Geometry check sheet. Reference: drawing and pictorial views, mm from the part's lowest x, y, z. A direction names the side the tool comes from. Round coordinates to 2 decimals unless told otherwise and drop trailing zeros. Loops run counter-clockwise (first coordinate to the right, second up) from the corner with the lowest first, then second, coordinate; pieces in that order, holes last. Notation, with made-up numbers: (37, -10) - (51, -10) arc R34 cw to (51, 20) - close; hole circle Ø2 at (33, 76.5). An arc over 180 degrees is marked (long way). Return JSON: item names as keys, results as strings.
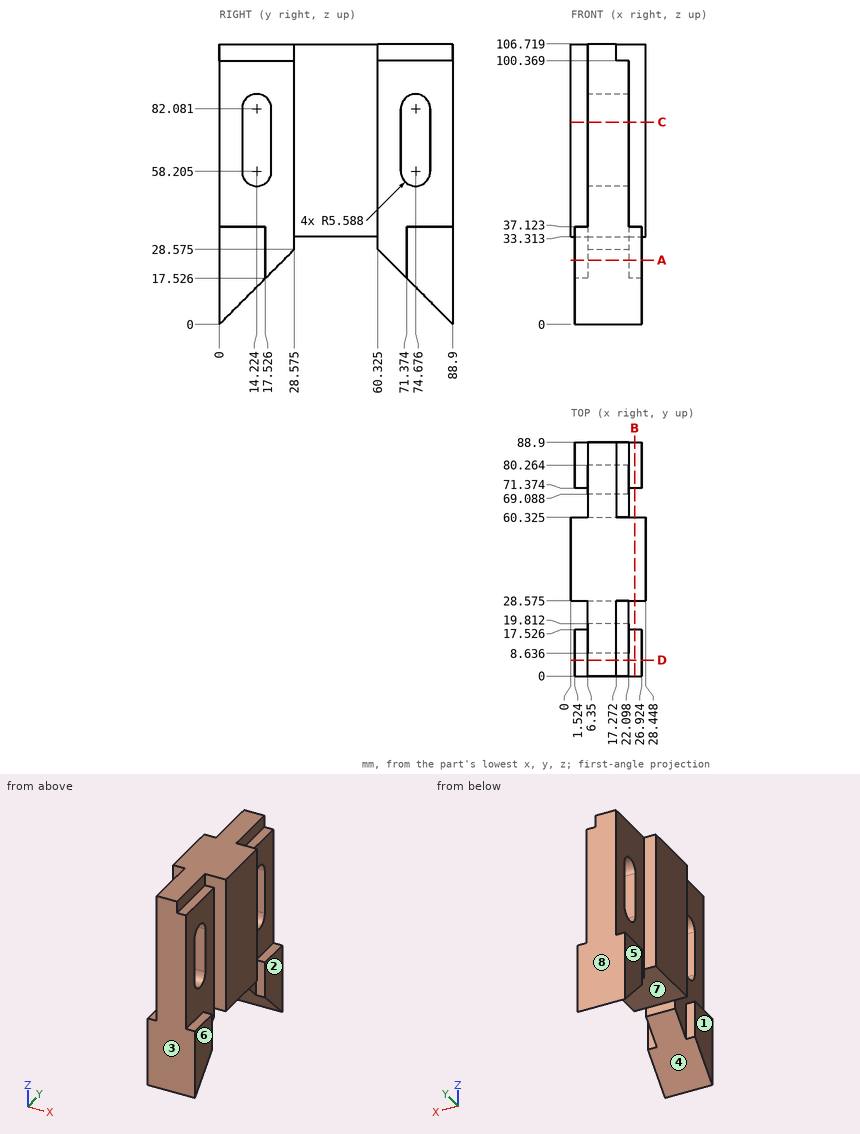
Q1. Sectioned sample at A-A (z = 24.5). Enter the section's corners in (x, y), plus the area to 3 significant figures.
Answer key:
{"outline": "(1.52, 0) - (26.92, 0) - (26.92, 17.53) - (22.1, 17.53) - (22.1, 24.5) - (6.35, 24.5) - (6.35, 17.53) - (1.52, 17.53) - close; (1.52, 71.37) - (6.35, 71.37) - (6.35, 64.4) - (22.1, 64.4) - (22.1, 71.37) - (26.92, 71.37) - (26.92, 88.9) - (1.52, 88.9) - close", "area": "1,110 mm²"}
Q2. Sectioned sample at C-C (z = 77). Enter the section's corners in (x, y) (3 decimals).
Answer key:
{"outline": "(0, 28.575) - (6.35, 28.575) - (6.35, 19.812) - (22.098, 19.812) - (22.098, 28.575) - (28.448, 28.575) - (28.448, 60.325) - (22.098, 60.325) - (22.098, 69.088) - (6.35, 69.088) - (6.35, 60.325) - (0, 60.325) - close; (6.35, 0) - (22.098, 0) - (22.098, 8.636) - (6.35, 8.636) - close; (6.35, 80.264) - (22.098, 80.264) - (22.098, 88.9) - (6.35, 88.9) - close"}
Q3. Sectioned sample at B-B (x = 24.25). Enter the section's corners in (y, z) (3 decimals), plus the area to 3 significant figures.
Answer key:
{"outline": "(0, 0) - (17.526, 17.526) - (17.526, 37.123) - (0, 37.123) - close; (28.575, 33.313) - (60.325, 33.313) - (60.325, 106.719) - (28.575, 106.719) - close; (71.374, 17.526) - (88.9, 0) - (88.9, 37.123) - (71.374, 37.123) - close", "area": "3,320 mm²"}
Q4. Scan lines: probe 1 along Y at (x, z) = (15, 71.5); probe 2 along X at (y, z) = (20.5, 88); probe 3 along Y at (x, z) = (11.75, 56.5). Record each from-to range of solid material in increasing order. Write a range as [from, to].
Answer key:
{"probe 1": "y = [0, 8.64], [19.81, 69.09], [80.26, 88.9]", "probe 2": "x = [6.35, 22.1]", "probe 3": "y = [0, 8.9], [19.55, 69.35], [80, 88.9]"}
Q5. Depth check by flat-ended pin: P1, Ø1, axis at y = 10, z = 89, coming from the +X side; P2, Ø7, axis at y = 78.5, z = 104, coming from the +X side; P3, Ø14, axis at y = 10.5, z = 14, coming from the -X side. Enter the tip coordinate at first touch or a pass-through.
Answer key:
{"P1": "stops at x = 22.1", "P2": "stops at x = 17.27", "P3": "stops at x = 1.52"}
Q6. Tool access check on the marked faces 1, 2, 3, 4 and 5. Record the directions out of +Z, -Z, +X, -X, +Y, -Y that give a thin tool (end or side, any length) a straight path to the whole face; none if there is none.
Answer key:
{"face 1": "+Z, -Z, -X, -Y", "face 2": "+Z, -Z, +X, +Y", "face 3": "+Z, -Z, +X, -X, -Y", "face 4": "-Z, +X, -X", "face 5": "+Z, -Z, -X, +Y"}
Q7. Draft check along Y on the marked faces 6, 7 and 8. Enter one of: released by +Y, released by -Y, zero draft, split by the parting line, or undercut.
Answer key:
{"face 6": "zero draft", "face 7": "undercut", "face 8": "released by +Y"}
Q8. Sectioned sample at D-D (y = 6). Enter the section's corners in (x, z).
Answer key:
{"outline": "(1.52, 6) - (26.92, 6) - (26.92, 37.12) - (22.1, 37.12) - (22.1, 100.37) - (17.27, 100.37) - (17.27, 106.72) - (6.35, 106.72) - (6.35, 37.12) - (1.52, 37.12) - close"}
